from build123d import *

# Parameters (mm, degrees)
SKETCH1_W           = 25.4
SKETCH1_H           = 21.336
SKETCH1_R           = 3.9624
BOSS_EXTRUDE1_DEPTH = 44.069
SKETCH3_R           = 2.286
CUT_EXTRUDE2_DEPTH  = 3.175


with BuildPart() as part:
    # Sketch1 → Boss-Extrude1 (new body)
    with BuildSketch(Plane(origin=(0, 0, 0), x_dir=(1, 0, 0), z_dir=(0, 1, 0))):
        with Locations((12.7, -10.668)):
            Rectangle(SKETCH1_W, SKETCH1_H)
        with Locations(Location((12.7, -10.668, 0), (0, 0, 270))):
            Circle(SKETCH1_R, mode=Mode.SUBTRACT)
    extrude(amount=BOSS_EXTRUDE1_DEPTH)

    # Sketch3 → Cut-Extrude2 (cut)
    with BuildSketch(Plane.ZY):
        with Locations((16.1798, 32.258)):
            Circle(SKETCH3_R)
        with Locations((5.1562, 19.558)):
            Circle(SKETCH3_R)
    extrude(amount=-CUT_EXTRUDE2_DEPTH, mode=Mode.SUBTRACT)


solid = part.part
Verification items for the finished model (mm, model axes). A direction names the side the tool comes from. Give positions to 0.01 mm unless a question says otherwise; leave off trailing zeros. Write each loop counter-clockwise with the first axis right and the second up, starting at its lowest first coordinate (ties: lowest second). Pieces come first, ordered by that corner, then holes. Notation, with made-up numbers: M 53.5,31.25 L 71.5,31.25 A16 ccw 71.5,58.25 Z; hole C -7.5,75.25 d7. An arc over 180 degrees is marked long. Put each result on its own line as item: value. Start each with the question number.
1. Section check C-C (y = 37). Record the cut outline in (x, z), and give its area (3 significant figures).
2. Section check A-A (x = 12.7). Record the cut outline in (y, z), and give its area (3 significant figures).
3. Set-up check for faces 1 (the face through (13, 22, 21.336)), 2 (the face through (3.175, 20, 5)): record each of +Z, -Z, +X, -X, +Y, -Y from which the full face is reachable in a straight line by a thin tool's end or side.
4. Section check B-B (z = 8.5). Record the cut outline in (x, y), and give its area (3 significant figures).
5. Draft check along Y on faces 3 (the face through (25.4, 22, 11)), 4 (the face through (13, 0, 6)), 5 (the face through (1.565, 18.682, 7.268)), 6 (the face through (1.57, 32.94, 18.36)). Enter one of: +Y half, -Y half, draft (parallel to the pull), parting line (faces both ways), or undercut.
6. Scan lines: line 1 along X through (y, z) = (14.5, 13); line 2 along X through (y, z) = (35, 9); line 3 along Z through (x, y) = (13.75, 38.5). Record each from-to range of solid material in increasing order. Write a range as [from, to].
Answer list:
1. outline: M 0,0 L 25.4,0 L 25.4,21.34 L 0,21.34 Z; hole C 12.7,10.67 d7.92
1. area: 493 mm2
2. outline: M 0,0 L 44.07,0 L 44.07,6.71 L 0,6.71 Z; M 0,14.63 L 44.07,14.63 L 44.07,21.34 L 0,21.34 Z
2. area: 591 mm2
3. face 1: +Z, +X, -X, +Y, -Y
3. face 2: -X
4. outline: M 0,0 L 9.38,0 L 9.38,44.07 L 0,44.07 Z; M 16.02,0 L 25.4,0 L 25.4,44.07 L 16.02,44.07 Z
4. area: 827 mm2
5. face 3: draft
5. face 4: -Y half
5. face 5: undercut
5. face 6: undercut
6. line 1: [0, 9.5], [15.9, 25.4]
6. line 2: [0, 9.11], [16.29, 25.4]
6. line 3: [0, 6.85], [14.49, 21.34]
